Autodesk Inventor part; units mm, degrees
ref_plane "Work Plane1" through (25.4, 0, 0) normal (-1, 0, 0) x (0, 0, 1)
ref_plane "YZ Plane" through (0, 0, 0) normal (1, 0, 0) x (0, 1, 0)
ref_plane "XZ Plane" through (0, 0, 0) normal (0, 1, 0) x (-1, 0, 0)
sketch "Sketch1" plane through (0, 0, 0) normal (0, 0, 1) x (1, 0, 0)
  line L0 (0, 0) -> (50.8, 0) construction
  line L1 (0, 82.55) -> (0, 76.2)
  line L2 (0, 76.2) -> (50.8, 76.2)
  line L3 (50.8, 76.2) -> (50.8, 82.55)
  line L4 (50.8, 82.55) -> (0, 82.55)
  dimension "d1" = 50.8
  dimension "d7" = 76.2
  dimension "d8" = 6.35
revolve "Revolution1" add sketch "Sketch1" angle 360 about axis through (0, 0, 0) along (1, 0, 0)
sketch "Sketch2" plane through (50.8, 0, 0) normal (1, 0, 0) x (0, 0, -1)
  circle A0 centre (0, 0) radius 82.55
  circle A1 centre (0, 0) radius 76.2
extrude "Extrusion1" add sketch "Sketch2" along normal blind 6.35 contours A0 | A1
sketch "Sketch3" plane through (50.8, 0, 0) normal (-1, 0, 0) x (0, 0, 1)
  point P0 (0, 0)
  point P1 (0, 50.8)
  point P2 (0, 0)
  dimension "d9" = 50.8
hole "Hole1" at (50.8, 50.8, 0) at (50.8, 0, 0) direction (1, 0, 0) diameter 6.858 end through all
pattern_circular "Circular Pattern1" count 5 over 360 about axis through (25.4, 0, 0) along (1, 0, 0) of "Hole1"
ref_plane "Work Plane1" through (25.4, 0, 0) normal (-1, 0, 0) x (0, 0, 1)
sketch "Sketch5" plane through (25.4, 0, 0) normal (-1, 0, 0) x (0, 0, 1)
  circle A0 centre (0, 0) radius 76.2
  circle A1 centre (0, 0) radius 82.55
  circle A2 centre (48.3137, 15.6981) radius 3.429
  circle A3 centre (29.8595, -41.0981) radius 3.429
  circle A4 centre (0, 50.8) radius 3.429 construction
  circle A5 centre (0, 0) radius 3.429
  circle A6 centre (0, 0) radius 76.2
  circle A7 centre (0, 50.8) radius 3.429 construction
  circle A8 centre (0, 50.8) radius 9.525 construction
  line L0 (0, 60.325) -> (49.1356, 60.325) construction
  line L1 (49.1356, 60.325) -> (49.1356, 41.275) construction
  line L2 (49.1356, 41.275) -> (0, 41.275) construction
  line L3 (0, 41.275) -> (0, 60.325) construction
  circle A9 centre (0, 50.8) radius 50.4056 construction
  circle A10 centre (0, 0) radius 76.2
  arc A11 (49.9526, 57.5428) -> (47.5712, 67.4647) centre (0, 50.8) ccw
  line L4 (-9.525, 50.8) -> (-9.525, 81.9986) construction
  circle A12 centre (0, 0) radius 76.2
  line L5 (-9.525, 75.6023) -> (-9.525, 81.9986)
  arc A13 (49.9526, 57.5428) -> (-9.525, 75.6023) centre (0, 0) ccw
  arc A14 (47.5712, 67.4647) -> (-9.525, 81.9986) centre (0, 0) ccw
  point P0 (49.9526, 57.5428)
  dimension "d27" = 19.05
  dimension "d28" = 19.05
  dimension "d29" = 49.1356
  dimension "d30" = 100.8113
  dimension "d31" = 82.55
extrude "Extrusion2" cut sketch "Sketch5" along normal mid plane 9.525 contours A0 L5 A1 A11 picked at (-1.9672, 80.2341)
pattern_circular "Circular Pattern2" count 5 over 360 about axis through (291.1792, 0, 0) along (-1, 0, 0) of "Extrusion2"
equation "\"d1\" = wheelDepth"
equation "\"d7\" = wheelR"
equation "\"d8\" = wheelThickness"
equation "\"d10\" = smallHoles"
equation "\"d27\" = swivelBaseDiameter"
equation "\"d28\" = d27"
equation "\"d29\" = swivelLegLength"
equation "\"d31\" = wheelR + wheelThickness"
equation "\"d32\" = 0.5 * swivelLegThickness"
equation "\"gearShaft\" = 6.35"
equation "\"largeGear\" = 38.1"
equation "\"smallGear\" = 12.7"
equation "\"wheelR\" = 76.2"
equation "\"wheelThickness\" = 6.35"
equation "\"wheelDepth\" = 50.8"
equation "\"mainHole\" = 6.858"
equation "\"smallHoles\" = 6.858"
equation "\"farFromCenter\" = 50.8"
equation "\"smallGearLength\" = 50.8"
equation "\"mainGearLength\" = 76.2"
equation "\"gearThickness\" = 6.35"
equation "\"mainGear\" = 38.1"
equation "\"d20\" = -0.5 * wheelDepth"
equation "\"swivelBaseDiameter\" = 19.05"
equation "\"swivelLegExtentions\" = 19.05"
equation "\"swivelLegLength\" = 49.13565"
equation "\"swivelLegThickness\" = 19.05"
properties part number "Wheel1"
Work out the finished part from the listing and answer in its coordinate system (mm). A direction names the side the tool comes from. Round coordinates to 2 decimals unless told otherwise and drop trailing zeros. Write each loop counter-clockwise with the first axis right and the second up, starting at its lowest first coordinate (ties: lowest second). Pieces come first, ordered by that corner, then holes. Notation, with made-up numbers: (85, -18) - (121, -18) arc R22 ccw to (121, 14) - close; hole circle Ø4 at (22.25, -24.75). An arc over 180 degrees is marked (long way). Return JSON: item names as keys, results as strings. Group by question number.
Q1. Each of these flat-tipped pins is pushed along its axis until it touches: pin 1 Ø10 at (x, y) = (28, -40) entering from -Z; pin 2 Ø12.5 at (y, z) = (74, 7) entering from -X; pin 3 Ø4 at (x, y) = (7, 30.5) entering from +Z; pin 4 Ø1 at (y, z) = (57.5, -60) entering from +X. Where does it stop, or does it pass through?
Q2. The mould has two halves that part along Z. Classify faces 1 (the flat face through (20.638, 42, -64)), 2 (the flat face through (25.467, 15.278, -77.844)), 3 (the cylindrical face through (25.467, -21.872, -76.454)): released by +Z, released by -Z, zero draft, split by the parting line, or undercut.
Q3. Find the intervals of material crossed by L1, parallel to Y at x = 53, z = 0; L2, parallel to Y at x = 17.5, z = 0; L3, parallel to X at y = -34, z = -70, in increasing order.
Q4. The part is cut by section B-B on x = 26.5. Count the separate pieces of the cut face and the enclosed holes in it, then the cut area to 3 significant figures.
Q5. The part is cut by section C-C on z = 39. Write down the section's boundary in (x, y).
Q6. The part is cut by section D-D on y = -35. Write down the section's boundary in (x, z).
Q7. The part is cut by section A-A on y = 0. Write down the section's boundary in (x, z), then the cut area to 3 significant figures.
Q8. For faces 4 (the cylindrical face through (25.467, -79.471, -2.824)), 5 (the cylindrical face through (25.467, -27.244, 74.709)), 6 (the flat face through (25.467, 33.396, 71.958)), 7 (the flat face through (50.8, -16, 1)), 8 (the flat face through (25.467, -69.313, -38.586)), determine the directions among +Z, -Z, +X, -X, +Y, -Y from which every point of the face is accessible in a straight line to the end or side of a thin tool.
Solved:
{
 "1": {"pin 1": "z = -74.53", "pin 2": "x = 0", "pin 3": "z = 77.47", "pin 4": "through"},
 "2": {"face 1": "zero draft", "face 2": "released by +Z", "face 3": "undercut"},
 "3": {"L1": "-82.55 to -3.43, 3.43 to 47.37, 54.23 to 82.55", "L2": "-82.55 to -76.2, 76.2 to 82.55", "L3": "0 to 20.64, 30.16 to 57.15"},
 "4": {"separate pieces": "5", "enclosed holes": "0", "area": "1,190 mm²"},
 "5": {"outline": "(0, -72.76) - (20.64, -72.76) - (20.64, -65.46) - (0, -65.46) - close; (0, 65.46) - (20.64, 65.46) - (20.64, 72.76) - (0, 72.76) - close; (30.16, -72.76) - (57.15, -72.76) - (57.15, 72.76) - (30.16, 72.76) - (30.16, 65.46) - (50.8, 65.46) - (50.8, -65.46) - (30.16, -65.46) - close"},
 "6": {"outline": "(0, -74.76) - (20.64, -74.76) - (20.64, -67.69) - (0, -67.69) - close; (0, 67.69) - (50.8, 67.69) - (50.8, -67.69) - (30.16, -67.69) - (30.16, -74.76) - (57.15, -74.76) - (57.15, 74.76) - (0, 74.76) - close"},
 "7": {"outline": "(0, -82.55) - (57.15, -82.55) - (57.15, -3.43) - (50.8, -3.43) - (50.8, -76.2) - (0, -76.2) - close; (0, 76.2) - (20.64, 76.2) - (20.64, 82.55) - (0, 82.55) - close; (30.16, 76.2) - (50.8, 76.2) - (50.8, 3.43) - (57.15, 3.43) - (57.15, 82.55) - (30.16, 82.55) - close", "area": "1,590 mm²"},
 "8": {"face 4": "+Z, +Y", "face 5": "none", "face 6": "+Z", "face 7": "-X", "face 8": "-Z"}
}
